from build123d import *

# Parameters (mm, degrees)
BASE_EXTRUDE_DEPTH = 15.875
SKETCH3_R          = 1.397
CUT_EXTRUDE2_DEPTH = 12.7


with BuildPart() as part:
    # Sketch1 → Base-Extrude (new body, symmetric)
    with BuildSketch(Plane.XY):
        Polygon((6.35, 0), (-6.35, 0), (-3.816827491, 10.16), (-9.525, 10.16), (-9.525, 15.24), (9.525, 15.24), (9.525, 10.16), (3.816827491, 10.16), align=None)
    extrude(amount=BASE_EXTRUDE_DEPTH, both=True)

    # Sketch3 → Cut-Extrude2 (cut)
    with BuildSketch(Plane(origin=(0, 15.24, 0), x_dir=(-1, 0, 0), z_dir=(0, 1, 0))):
        Circle(SKETCH3_R)
    extrude(amount=-CUT_EXTRUDE2_DEPTH, mode=Mode.SUBTRACT)


solid = part.part
Read the model definition and answer for the solid it produces. Units are mm, in the model's axes. A direction names the side the tool comes from. Round coordinates to 2 decimals unless told otherwise and drop trailing zeros. Order: outer loops, then holes, each group sorted by start corner. A loop starts at its lowest first (then second) coordinate and runs counter-clockwise, first axis right, second up.
1) The mould has two halves that part along Y. Classify faces 5 (the face through (-7, 10.16, 0)), 6 (the face through (9.525, 13, 0)), 7 (the face through (2, 15.24, 0)): released by +Y, released by -Y, zero draft, split by the parting line, or undercut.
2) The part is cut by section A-A on z = -5.5. Write down the section's boundary in (x, y) (3 decimals).
3) For faces 1 (the face through (1.11, 8.98, -0.85)), 2 (the face through (0, 9, 15.875)), 3 (the face through (-5.1, 5.01, 0.22)), 4 (the face through (5.066, 5.151, 0.222)), determine the directions among +Z, -Z, +X, -X, +Y, -Y from which every point of the face is accessible in a straight line to the end or side of a thin tool.
4) The part is cut by section C-C on y = 9.75. Write down the section's boundary in (x, z) (3 decimals).
5) Straight lines are drawn through the part: L1, parallel to Z at x = 0, y = 8.75 (3 decimals); L2, parallel to Y at x = 8.25, z = -10; L3, parallel to X at y = 1.5, z = 14. For each, find the intervals that lie inside material, in ascending order.
6) The part is cut by section B-B on x = 0. Write down the section's boundary in (y, z) (3 decimals), plus the area to 3 significant figures.
7) Flat-ended cylindrical pins translate along their axes: pin 1 (3 mm diameter, centred on x = -5.5, z = -6.5, fed in from -Y); pin 2 (3 mm diameter, centred on x = 8, z = 7.5, fed in from -Y); pin 3 (1.7 mm diameter, centred on x = 0, z = 0, fed in from +Y). Find the tip coordinate at first contact, or state that the pin passes through.
8) The part is cut by section D-D on x = -5.25. Write down the section's boundary in (y, z) (3 decimals), plus the area to 3 significant figures.
Resolved:
1. face 5: undercut
1. face 6: zero draft
1. face 7: released by +Y
2. outline: (-9.525, 10.16) - (-3.817, 10.16) - (-6.35, 0) - (6.35, 0) - (3.817, 10.16) - (9.525, 10.16) - (9.525, 15.24) - (-9.525, 15.24) - close
3. face 1: +Y
3. face 2: +Z, +X, -X, +Y, -Y
3. face 3: +Z, -Z, -X
3. face 4: +Z, -Z, +X
4. outline: (-3.919, -15.875) - (3.919, -15.875) - (3.919, 15.875) - (-3.919, 15.875) - close; hole circle Ø2.794 at (0, 0)
5. L1: z = -15.875 to -1.397, 1.397 to 15.875
5. L2: y = 10.16 to 15.24
5. L3: x = -5.98 to 5.98
6. outline: (0, -15.875) - (15.24, -15.875) - (15.24, -1.397) - (2.54, -1.397) - (2.54, 1.397) - (15.24, 1.397) - (15.24, 15.875) - (0, 15.875) - close
6. area: 448 mm2
7. pin 1: stops at y = 0
7. pin 2: stops at y = 10.16
7. pin 3: stops at y = 2.54
8. outline: (0, -15.875) - (4.412, -15.875) - (4.412, 15.875) - (0, 15.875) - close; (10.16, -15.875) - (15.24, -15.875) - (15.24, 15.875) - (10.16, 15.875) - close
8. area: 301 mm2
